Input: part model. Units: mm. Frame: model coordinates. Round coordinates to 2 decimals unless told otherwise and drop trailing zeros. Loops run counter-clockwise (first coordinate to the right, second up) from the corner with the lowest first, then second, coordinate; pieces in that order, holes last.
(1) Line query: line 1 (Y direction, x = -48, z = 3.75); line 2 (X direction, y = 36, z = 2); line 3 (X direction, y = 34, z = 6). Output: solid intervals per line, ascending.
(2) Cut plane A-A, the plane z = 20.25. Output: boundary loops of the cut face in (x, y), and give its area (3 significant figures).
(3) First-contact query: pin 1 Ø2.5 at (x, y) = (-48, -9.5) entering from +Z. Flat tip, straight axial feed; report the tip coordinate or a pass-through.
from build123d import *

# Parameters (mm, degrees)
SKETCH2_W                                           = 38.1
SKETCH2_H                                           = 50.8
BOSS_EXTRUDE1_DEPTH                                 = 25.4
CBORE_FOR_6_BINDING_HEAD_MACHINE_SCREW1_D           = 3.7973
CBORE_FOR_6_BINDING_HEAD_MACHINE_SCREW1_CBORE_D     = 7.9375
CBORE_FOR_6_BINDING_HEAD_MACHINE_SCREW1_CBORE_DEPTH = 2.2098


with BuildPart() as part:
    # Sketch2 → Boss-Extrude1 (new body)
    with BuildSketch(Plane.XY):
        with Locations((-32.515060241, 13.847590361)):
            Rectangle(SKETCH2_W, SKETCH2_H)
    extrude(amount=BOSS_EXTRUDE1_DEPTH)

    # CBORE for #6 Binding Head Machine Screw1 (through all)
    with Locations(Plane(origin=(-47.755060241, 35.437590361, 25.4), x_dir=(1, 0, 0), z_dir=(0, 0, 1))):
        with Locations((0, 0), (30.48, 0), (0, -43.18), (30.48, -43.18)):
            CounterBoreHole(CBORE_FOR_6_BINDING_HEAD_MACHINE_SCREW1_D / 2, CBORE_FOR_6_BINDING_HEAD_MACHINE_SCREW1_CBORE_D / 2, CBORE_FOR_6_BINDING_HEAD_MACHINE_SCREW1_CBORE_DEPTH)


solid = part.part
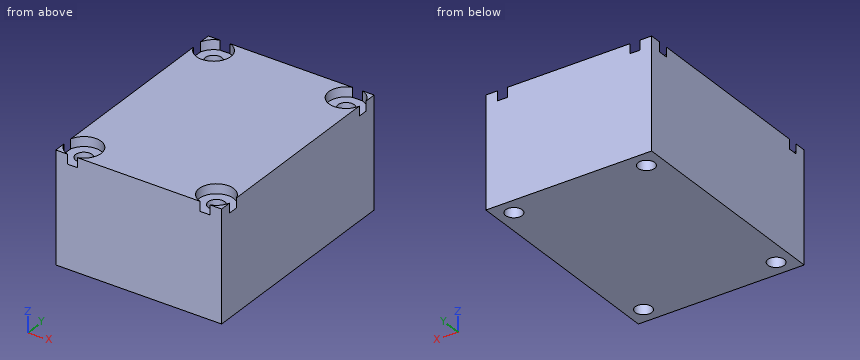
Reported:
1. line 1: y = -11.55 to -9.63, -5.86 to 33.55, 37.32 to 39.25
1. line 2: x = -51.57 to -49.57, -45.94 to -19.09, -15.46 to -13.47
1. line 3: x = -51.57 to -49, -46.51 to -18.52, -16.03 to -13.47
2. outline: (-51.57, -11.55) - (-13.47, -11.55) - (-13.47, 39.25) - (-51.57, 39.25) - close; hole circle Ø3.8 at (-47.76, -7.74); hole circle Ø3.8 at (-47.76, 35.44); hole circle Ø3.8 at (-17.28, -7.74); hole circle Ø3.8 at (-17.28, 35.44)
2. area: 1,890 mm2
3. pin 1: stops at z = 23.19
